```python
from build123d import *

# Parameters (mm, degrees)
EXTRUDE_1_DEPTH     = 33
SKETCH_2_R          = 10
EXTRUDE_2_DEPTH     = 25
SKETCH_3_R          = 4
CUT_EXTRUDE_1_DEPTH = 8
SKETCH_4_R          = 3.46188381
CUT_EXTRUDE_2_DEPTH = 25


with BuildPart() as part:
    # 草图1 → 凸台-拉伸1 (new body)
    with BuildSketch(Plane(origin=(0, 0, 0), x_dir=(1, 0, 0), z_dir=(0, 1, 0))):
        with BuildLine():
            Line((-16, 12), (-16, -12))
            ThreePointArc((-16, -12), (0, -20), (16, -12))
            Line((16, -12), (16, 12))
            ThreePointArc((16, 12), (0, 20), (-16, 12))
        make_face()
    extrude(amount=EXTRUDE_1_DEPTH)

    # 草图2 → 凸台-拉伸2 (add)
    with BuildSketch(Plane.XZ):
        with Locations(Location((0, 0, 0), (0, 0, 270))):
            Circle(SKETCH_2_R)
    extrude(amount=EXTRUDE_2_DEPTH)

    # 草图3 → 切除-拉伸1 (cut)
    with BuildSketch(Plane(origin=(0, 33, 0), x_dir=(1, 0, 0), z_dir=(0, 1, 0))):
        with Locations(Location((0, 0, 0), (0, 0, 270))):
            Circle(SKETCH_3_R)
    extrude(amount=-CUT_EXTRUDE_1_DEPTH, mode=Mode.SUBTRACT)

    # 草图4 → 切除-拉伸2 (cut)
    with BuildSketch(Plane.XZ.offset(25)):
        with Locations(Location((0, 0, 0), (0, 0, 270))):
            Circle(SKETCH_4_R)
    extrude(amount=-CUT_EXTRUDE_2_DEPTH, mode=Mode.SUBTRACT)


solid = part.part
```
Input: part model. Units: mm. Frame: model coordinates. A direction names the side the tool comes from. Give positions to 0.01 mm unless a question says otherwise; leave off trailing zeros. Loops run counter-clockwise (first coordinate to the right, second up) from the corner with the lowest first, then second, coordinate; pieces in that order, holes last. Notation, with made-up numbers: (55.25, -16.75) -> (74.25, -16.75) arc R10 cw to (74.25, -4.75) -> close; hole circle Ø9 at (-31.75, 42.25). An arc over 180 degrees is marked (long way). Use a Markdown table: item, result.
Q1. Section query B-B, the plane z = 0. Return the cut outline in (x, y), plus the area to 3 significant figures.
Entries:
| item | result |
|---|---|
| outline | (-16, 0) -> (-10, 0) -> (-10, -25) -> (-3.46, -25) -> (-3.46, 0) -> (3.46, 0) -> (3.46, -25) -> (10, -25) -> (10, 0) -> (16, 0) -> (16, 33) -> (4, 33) -> (4, 25) -> (-4, 25) -> (-4, 33) -> (-16, 33) -> close |
| area | 1,320 mm² |
Q2. Section query D-D, the plane y = 19. Return the cut outline in (x, z).
Entries:
| item | result |
|---|---|
| outline | (-16, -12) arc R20 ccw to (16, -12) -> (16, 12) arc R20 ccw to (-16, 12) -> close |
Q3. Access query for faces 1 (the flat face through (0, 25, 0)), 2 (the flat face through (0, 0, 0)), 3 (the flat face through (16, 16, 0)). Directions: +Z, -Z, +X, -X, +Y, -Y. A direction counts if a zero-diameter tool reaches every point of the face in a straight line with its end or side. Return the directions, or none.
Entries:
| item | result |
|---|---|
| face 1 | +Y |
| face 2 | -Y |
| face 3 | +Z, -Z, +X, +Y, -Y |
Q4. Section query C-C, the plane y = -9.5. Return the cut outline in (x, z), plus the area to 3 significant figures.
Entries:
| item | result |
|---|---|
| outline | circle Ø20 at (0, 0); hole circle Ø6.92 at (0, 0) |
| area | 277 mm² |
Q5. Ray query, probe 1 along X at (y, z) = (29.75, 0); probe 2 along X at (y, z) = (-14.75, 0); probe 3 along Y at (x, z) = (-7, -14). Return the intervals inside material, ascending. Write a range as from..to.
Entries:
| item | result |
|---|---|
| probe 1 | x = -16..-4, 4..16 |
| probe 2 | x = -10..-3.46, 3.46..10 |
| probe 3 | y = 0..33 |
Q6. Section query A-A, the plane x = 0. Return the cut outline in (y, z), plus the area to 3 significant figures.
Entries:
| item | result |
|---|---|
| outline | (-25, -10) -> (0, -10) -> (0, -20) -> (33, -20) -> (33, -4) -> (25, -4) -> (25, 4) -> (33, 4) -> (33, 20) -> (0, 20) -> (0, 10) -> (-25, 10) -> (-25, 3.46) -> (0, 3.46) -> (0, -3.46) -> (-25, -3.46) -> close |
| area | 1,580 mm² |
Q7. Pull-direction query (X, two-part tool) for faces 4 (the cylindrical face through (0, 16, 20)), 5 (the cylindrical face through (-3.38, -12.68, 0.75)), 6 (the flat face through (-16, 16, 0)); classes: pulls with the +X half, pulls with the -X half, needs draft (parallel to the pull), parting line crosses it, or undercut.
Entries:
| item | result |
|---|---|
| face 4 | parting line crosses it |
| face 5 | undercut |
| face 6 | pulls with the -X half |
Q8. First-contact query: P1, Ø12, axis at y = -17, z = -14, coming from the -X side; P2, Ø1, axis at x = 3, y = 4, coming from the +Z side; P3, Ø4, axis at y = -16, z = -7, coming from the -X side. Flat tips, straight axial feed; report the tip coordinate or a pass-through.
Entries:
| item | result |
|---|---|
| P1 | stops at x = -6 |
| P2 | stops at z = 19.84 |
| P3 | stops at x = -8.66 |
